Geometry: final body of the model. Coordinates: model frame, mm. A direction names the side the tool comes from. Coordinates: 2 decimals unless noted, no trailing zeros. Write each loop counter-clockwise with the first axis right and the second up, starting at its lowest first coordinate (ties: lowest second). Pieces come first, ordered by that corner, then holes. Notation, with made-up numbers: M 85.25,-29 L 139.25,-29 A19 cw 139.25,-6 Z; hole C -17.75,67 d10. An arc over 180 degrees is marked long. Write item = value, one per line. Start each with the question number.
Item 1: Section D-D on y = 19. Output: boundary loops of the cut face in (x, z).
Item 2: First-contact query: pin 1 Ø8 at (y, z) = (20.5, 17.5) entering from +X; pin 2 Ø12 at (x, z) = (-14, 24.5) entering from +Y; pin 3 Ø10 at (x, y) = (-17.5, 22) entering from -Z. Flat tips, straight axial feed; report the tip coordinate or a pass-through.
Item 3: Ray query, L1, parallel to Y at x = -28.35, z = 19; L2, parallel to X at y = 18, z = 2; L3, parallel to Y at x = -6.75, z = 17.5. Return the intervals inside material, ascending. Write a range as [from, to].
Item 4: Pull-direction query (X, two-part tool) for faces 1 (the flat face through (-7, 2, 5)), 2 (the flat face through (-27, 19, 15)), 3 (the flat face through (-13, 3, 19)); classes: +X half, -X half, draft (parallel to the pull), parting line (faces both ways), or undercut.
Item 5: Section A-A on z = 32. Output: boundary loops of the cut face in (x, y), plus the area to 3 significant figures.
Item 6: Section C-C on x = -4.5. Output: boundary loops of the cut face in (y, z), plus the area to 3 significant figures.
Item 7: Reachability of faces 4 (the cylindrical face through (-21, 2, 9)), 5 (the flat face through (-15, 0, 19)) from +Z, -Z, +X, -X, +Y, -Y: full face, straight path, thin tool, end or side. Return the list, or none.
Item 8: Section B-B on z = 19. Output: boundary loops of the cut face in (x, y), plus the area to 3 significant figures.
Autodesk Inventor part; units mm, degrees
ref_plane "YZ Plane" through (0, 0, 0) normal (1, 0, 0) x (0, 1, 0)
ref_plane "XZ Plane" through (0, 0, 0) normal (0, 1, 0) x (-1, 0, 0)
ref_plane "XY Plane" through (0, 0, 0) normal (0, 0, 1) x (1, 0, 0)
sketch "Sketch1" plane through (0, 0, 0) normal (0, 1, 0) x (-1, 0, 0)
  line L0 (0, 0) -> (30, 0)
  line L1 (30, 0) -> (30, 38)
  line L2 (30, 38) -> (0, 38)
  line L3 (0, 38) -> (0, 0)
  dimension "d0" = 38
  dimension "d1" = 30
extrude "Extrusion1" add sketch "Sketch1" along normal blind 3
sketch "Sketch2" plane through (0, 3, 0) normal (0, 1, 0) x (1, 0, 0)
  line L0 (-30, 0) -> (-30, -38)
  line L1 (0, 0) -> (-30, 0)
  line L2 (-30, -38) -> (-27, -38)
  line L3 (-27, -38) -> (-27, 0)
  line L4 (-27, 0) -> (-30, 0)
  line L5 (-30, 0) -> (-30, -38)
  dimension "d4" = 3
extrude "Extrusion2" add sketch "Sketch2" along normal blind 27
sketch "Sketch3" plane through (-27, 3, 38) normal (1, 0, 0) x (0, 0, -1)
  circle A0 centre (19, 10.5) radius 6.5
  line L0 (38, 27) -> (0, 27)
  point P0 (38, -3)
  dimension "d7" = 13
  dimension "d8" = 16.5
extrude "Extrusion3" cut sketch "Sketch3" against normal up to surface (3 mm away)
sketch "Sketch4" plane through (0, 3, 0) normal (0, 1, 0) x (1, 0, 0)
  line L0 (0, 0) -> (-30, 0)
  line L1 (-27, -38) -> (-27, 0)
  line L2 (-27, -19) -> (0, -19) construction
  line L3 (-5.5, -35) -> (-5.5, -30.5) construction
  line L4 (-4, -35) -> (-4, -30.5)
  line L5 (-7, -30.5) -> (-7, -35)
  arc A0 (-7, -35) -> (-4, -35) centre (-5.5, -35) ccw
  arc A1 (-4, -30.5) -> (-7, -30.5) centre (-5.5, -30.5) ccw
  line L6 (-27, -38) -> (0, -38)
  line L7 (-5.5, -7.5) -> (-5.5, -3) construction
  line L8 (-7, -7.5) -> (-7, -3)
  line L9 (-4, -3) -> (-4, -7.5)
  arc A2 (-7, -7.5) -> (-4, -7.5) centre (-5.5, -7.5) ccw
  arc A3 (-4, -3) -> (-7, -3) centre (-5.5, -3) ccw
  line L10 (0, -38) -> (0, 0)
  line L11 (-4, -3) -> (-21, -3) construction
  line L12 (-21, -3) -> (-21, -7.5) construction
  line L13 (-22.5, -3) -> (-22.5, -7.5)
  line L14 (-19.5, -7.5) -> (-19.5, -3)
  arc A4 (-19.5, -3) -> (-22.5, -3) centre (-21, -3) ccw
  arc A5 (-22.5, -7.5) -> (-19.5, -7.5) centre (-21, -7.5) ccw
  line L15 (-21.1462, -34.8538) -> (-21.1462, -30.3538) construction
  line L16 (-22.7923, -34.8538) -> (-22.7923, -30.3538)
  line L17 (-19.5, -30.3538) -> (-19.5, -34.8538)
  arc A6 (-22.7923, -34.8538) -> (-19.5, -34.8538) centre (-21.1462, -34.8538) ccw
  arc A7 (-19.5, -30.3538) -> (-22.7923, -30.3538) centre (-21.1462, -30.3538) ccw
  point P0 (-5.5, -32.75)
  point P1 (-5.5, -5.25)
  point P2 (-21, -5.25)
  point P3 (-21.1462, -32.6038)
  dimension "d11" = 1.5
  dimension "d12" = 7.5
  dimension "d13" = 3
  dimension "d14" = 1.5
  dimension "d15" = 3
  dimension "d16" = 7.5
  dimension "d17" = 4
  dimension "d18" = 17
  dimension "d19" = 3
  dimension "d20" = 7.5
  dimension "d21" = 1.5
extrude "Extrusion4" cut sketch "Sketch4" against normal through all contours A0 L5 A1 L4 | L8 A3 L9 A2 | A4 L14 A5 L13 | L16 A7 L17 A6
equation "\"d14\" = d11"
equation "\"d15\" = d13"
equation "\"d16\" = d12"
equation "\"d19\" = d13"
properties part number "Big Motor Bracket"
Responses:
q1.outline = M -30,0 L -27,0 L -27,15.54 L -30,15.54 Z; M -30,22.46 L -27,22.46 L -27,38 L -30,38 Z
q2.pin_1 = -27
q2.pin_2 = 3
q2.pin_3 = through
q3.L1 = [0, 7], [20, 30]
q3.L2 = [-30, -27]
q3.L3 = [0, 3]
q4.face_1 = undercut
q4.face_2 = +X half
q4.face_3 = draft
q5.outline = M -30,0 L -22.79,0 L -22.79,3 L -27,3 L -27,30 L -30,30 Z; M -19.5,0 L -7,0 L -7,3 L -19.5,3 Z; M -4,0 L 0,0 L 0,3 L -4,3 Z
q5.area = 152 mm²
q6.outline = M 0,0 L 3,0 L 3,1.88 L 0,1.88 Z; M 0,8.62 L 3,8.62 L 3,29.38 L 0,29.38 Z; M 0,36.12 L 3,36.12 L 3,38 L 0,38 Z
q6.area = 73.6 mm²
q7.face_4 = +Y, -Y
q7.face_5 = +Z, -Z, +X, -X, -Y
q8.outline = M -30,0 L 0,0 L 0,3 L -27,3 L -27,7 L -30,7 Z; M -30,20 L -27,20 L -27,30 L -30,30 Z
q8.area = 132 mm²
